Part model, mm, in its own coordinate system. Face numbers are marked on the shaded views. A direction names the side the tool comes from. Round coordinates to 2 decimals unless told otherwise and drop trailing zeros. Loops run counter-clockwise (first coordinate to the right, second up) from the corner with the lowest first, then second, coordinate; pieces in that order, holes last. Notation, with made-up numbers: (44.25, 11.25) - (58.25, 11.25) arc R25 ccw to (58.25, 43.25) - close; hole circle Ø4 at (22, -6). An arc over 180 degrees is marked (long way). Write each question's results on one line, items separated by ' | '. Start each with the question number.
(1) Cut at D-D, the plane y = -28.5. List the corners of the cut face in (x, z), then the cut area to 3 significant figures.
(2) Mould opens along Z. For the marked faces 1, 2 and 3 say: released by +Z, released by -Z, zero draft, split by the parting line, or undercut.
(3) Cut at B-B, the plane y = -55. List the corners of the cut face in (x, z) (3 decimals).
(4) Cut at A-A, the plane x = 0. List the corners of the cut face in (y, z).
(5) Flat gauge pins, fed straight in: P1, Ø10, axis at x = 0, y = -59.98, coming from the +Z side; P2, Ø24, axis at x = -4.5, y = -45.5, coming from the -Z side; P3, Ø20.5, axis at y = 7, z = 11.5, coming from the +X side; P4, Ø10, axis at x = -15.5, z = -25, coming from the -Y side. Where does each tip first touch, or does it go through?
(6) Tool access for the marked faces 4, 5, 6 and 7: list every direction of +Z, -Z, +X, -X, +Y, -Y with a clear straight run to the whole face (end or side of a thin tool).
(7) Cut at C-C, the plane z = 18.5. List the corners of the cut face in (x, y).
(8) Drill centre lines: L1, parallel to Y at x = 0, z = -29; L2, parallel to Z at x = -27, y = -59; L3, parallel to X at y = 2, z = 32. Where is each one in solid material? Low to high.
from build123d import *

# Parameters (mm, degrees)
SALIENTE_EXTRUIR1_DEPTH = 38.1
SALIENTE_EXTRUIR2_DEPTH = 34.29
CROQUIS3_R              = 39.658757808
CORTAR_EXTRUIR1_DEPTH   = 12.7
CROQUIS4_R              = 6.35
CORTAR_EXTRUIR2_DEPTH   = 75.93


with BuildPart() as part:
    # Croquis1 → Saliente-Extruir1 (new body, symmetric)
    with BuildSketch(Plane(origin=(0, 0, 0), x_dir=(0, 0, -1), z_dir=(1, 0, 0))):
        Polygon((-40.64, 20.319999995), (-36.486122257, -20.319999995), (0, -20.319999995), (36.486122257, -20.319999995), (40.64, 20.319999995), align=None)
    extrude(amount=SALIENTE_EXTRUIR1_DEPTH, both=True)

    # Croquis2 → Saliente-Extruir2 (add, symmetric)
    with BuildSketch(Plane.XY):
        with BuildLine():
            Line((35.223664747, -20.319999995), (31.348920302, -35.687560492))
            ThreePointArc((31.348920302, -35.687560492), (0, -99.63751561), (-31.348920302, -35.687560492))
            Line((-31.348920302, -35.687560492), (-35.223664747, -20.319999995))
            Line((-35.223664747, -20.319999995), (35.223664747, -20.319999995))
        make_face()
    extrude(amount=SALIENTE_EXTRUIR2_DEPTH, both=True)

    # Croquis3 → Cortar-Extruir1 (cut, symmetric)
    with BuildSketch(Plane.XY):
        with Locations((0, -59.978757803)):
            Circle(CROQUIS3_R)
    extrude(amount=CORTAR_EXTRUIR1_DEPTH, both=True, mode=Mode.SUBTRACT)

    # Croquis4 → Cortar-Extruir2 (cut, through all)
    with BuildSketch(Plane.XY.offset(34.29)):
        with Locations((0, -59.978757803)):
            Circle(CROQUIS4_R)
    extrude(amount=-CORTAR_EXTRUIR2_DEPTH, mode=Mode.SUBTRACT)


solid = part.part
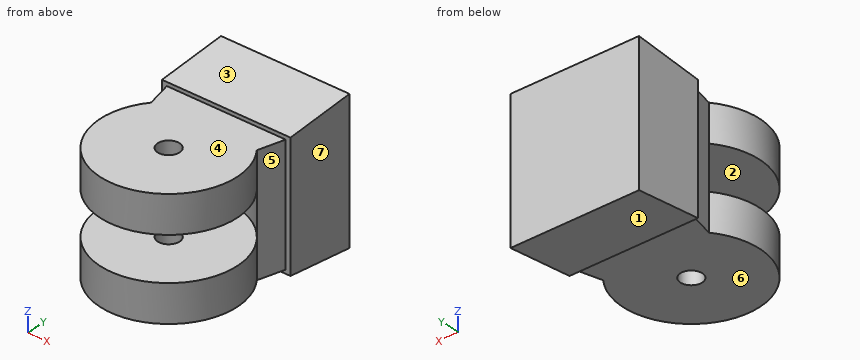
A:
1) outline: (-33.16, -34.29) - (33.16, -34.29) - (33.16, 34.29) - (-33.16, 34.29) - close; hole (-24.12, -12.7) - (24.12, -12.7) - (24.12, 12.7) - (-24.12, 12.7) - close | area: 3,320 mm2
2) face 1: released by -Z | face 2: undercut | face 3: released by +Z
3) outline: (-39.345, -34.29) - (-3.941, -34.29) - (-3.941, -12.7) - (-39.345, -12.7) - close; (-39.345, 12.7) - (-3.941, 12.7) - (-3.941, 34.29) - (-39.345, 34.29) - close; (3.941, -34.29) - (39.345, -34.29) - (39.345, -12.7) - (3.941, -12.7) - close; (3.941, 12.7) - (39.345, 12.7) - (39.345, 34.29) - (3.941, 34.29) - close
4) outline: (-99.64, -34.29) - (-66.33, -34.29) - (-66.33, -12.7) - (-99.64, -12.7) - close; (-99.64, 12.7) - (-66.33, 12.7) - (-66.33, 34.29) - (-99.64, 34.29) - close; (-53.63, -34.29) - (-20.32, -34.29) - (-20.32, -36.49) - (20.32, -40.64) - (20.32, 40.64) - (-20.32, 36.49) - (-20.32, 34.29) - (-53.63, 34.29) - (-53.63, 12.7) - (-20.32, 12.7) - (-20.32, -12.7) - (-53.63, -12.7) - close
5) P1: through | P2: z = -34.29 | P3: x = 38.1 | P4: y = -98.22
6) face 4: +Z, +X, -X, -Y | face 5: +Z, -Z, +X | face 6: -Z, +X, -X, -Y | face 7: +Z, -Z, +X, +Y
7) outline: (-38.1, -20.32) - (-35.22, -20.32) - (-31.35, -35.69) arc R39.66 ccw (long way) to (31.35, -35.69) - (35.22, -20.32) - (38.1, -20.32) - (38.1, 20.32) - (-38.1, 20.32) - close; hole circle Ø12.7 at (0, -59.98)
8) L1: -99.64 to -66.33, -53.63 to 20.32 | L2: -34.29 to -12.7, 12.7 to 34.29 | L3: -38.1 to 38.1
